```python
from build123d import *

# Parameters (mm, degrees)
F0_W      = 153.103292
F0_H      = 98.334714
F1_DEPTH  = 50.8
F2_R      = 44.312838
F2_R_2    = 37.577791
F3_DEPTH  = 25.4
F3_FACE_R = 37.577791
F4_DEPTH  = 76.2


with BuildPart() as f1:
    # F0 (on Front) → F1 (new body)
    with BuildSketch(Plane.XZ):
        Rectangle(F0_W, F0_H)
    extrude(amount=F1_DEPTH)

    # F2 (on face) → F3 (join)
    with BuildSketch(Plane.XZ.offset(50.8)):
        Circle(F2_R)
        Circle(F2_R_2, mode=Mode.SUBTRACT)
    extrude(amount=F3_DEPTH)

    # F3_face (on face) → F4 (cut)
    with BuildSketch(Plane.XZ.offset(50.8)):
        Circle(F3_FACE_R)
    extrude(amount=-F4_DEPTH, mode=Mode.SUBTRACT)


solid = f1.part
```
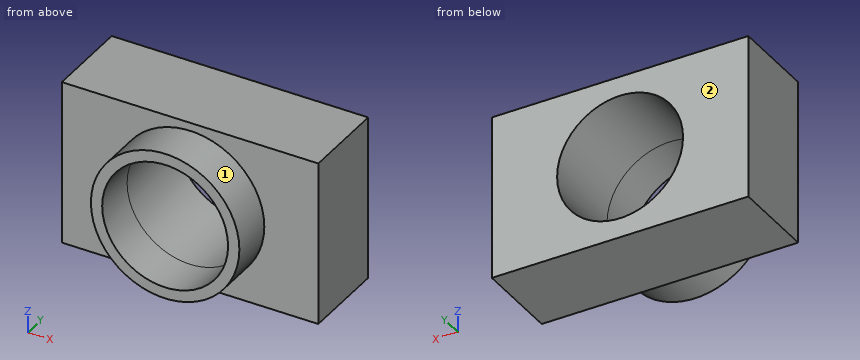
Design review of the part built by this model. Coordinates are the model's own, in mm. Face numbers are marked on the shaded views. A direction names the side the tool comes from. Coordinates: 2 decimals unless noted, no trailing zeros. Order: outer loops, then holes, each group sorted by start corner. A loop starts at its lowest first (then second) coordinate and runs counter-clockwise, first axis right, second up. Notation, with made-up numbers: (-18.5, -31.75) - (-1.5, -31.75) arc R25 cw to (-1.5, 7.25) - close; hole circle Ø3 at (-22, -18). An arc over 180 degrees is marked (long way). Answer in a Markdown table with one row per item.
(1) Wall thickness on line 1 along Z through (x, y) = (0, -57); line 2 along Z through (x, y) = (0, -16); line 3 along X through (y, z) = (-42, 4): over which ranges is each line inside the solid? List them lowest first. Write a range as from..to.
Checked values:
| item | result |
|---|---|
| line 1 | -44.31..-37.58, 37.58..44.31 |
| line 2 | -49.17..-37.58, 37.58..49.17 |
| line 3 | -76.55..-37.36, 37.36..76.55 |
(2) Consider section B-B on z = 0. State the section outline as (x, y) points, plus the area to 3 significant figures.
Checked values:
| item | result |
|---|---|
| outline | (-76.55, -50.8) - (-44.31, -50.8) - (-44.31, -76.2) - (-37.58, -76.2) - (-37.58, 0) - (-76.55, 0) - close; (37.58, -76.2) - (44.31, -76.2) - (44.31, -50.8) - (76.55, -50.8) - (76.55, 0) - (37.58, 0) - close |
| area | 4,300 mm^2 |
(3) Consider section A-A on x = 0. State the section outline as (y, z) points.
Checked values:
| item | result |
|---|---|
| outline | (-76.2, -44.31) - (-50.8, -44.31) - (-50.8, -49.17) - (0, -49.17) - (0, -37.58) - (-76.2, -37.58) - close; (-76.2, 37.58) - (0, 37.58) - (0, 49.17) - (-50.8, 49.17) - (-50.8, 44.31) - (-76.2, 44.31) - close |
(4) For the marked faces 1 and 2, list the 3-axis set-ups (+Z, -Z, +X, -X, +Y, -Y) from which the entire face can be reached by the end or side of a thin tool; tool diameter is ignored.
Checked values:
| item | result |
|---|---|
| face 1 | -Y |
| face 2 | +Z, -Z, +X, -X, +Y |
(5) Consider section C-C on y = -14. State the section outline as (x, z) points, plus the area to 3 significant figures.
Checked values:
| item | result |
|---|---|
| outline | (-76.55, -49.17) - (76.55, -49.17) - (76.55, 49.17) - (-76.55, 49.17) - close; hole circle Ø75.16 at (0, 0) |
| area | 10,600 mm^2 |
(6) Consider section D-D on z = -40. State the section outline as (x, y) points.
Checked values:
| item | result |
|---|---|
| outline | (-76.55, -50.8) - (-19.07, -50.8) - (-19.07, -76.2) - (19.07, -76.2) - (19.07, -50.8) - (76.55, -50.8) - (76.55, 0) - (-76.55, 0) - close |
(7) Clearance check with a flat-ended pin moving along its axis: pin 1 (2 mm diameter, centred on x = -41.5, z = -25.5, fed in from -Y). State where the tip first meets the part, or that it passes through.
Checked values:
| item | result |
|---|---|
| pin 1 | y = -50.8 |
